CAD build for the part. Positions are in the model's coordinates, mm. Round coordinates to 2 decimals unless told otherwise and drop trailing zeros. Put each result on its own line as item: value. Start each with the question number.
Item 1: Mould opens along Z. For faces 1 (the flat face through (-6, 148, 10)), 2 (the cylindrical face through (0.54, 147.74, 2.44)), 3 (the flat face through (10, 148, 6)) say: released by +Z, released by -Z, zero draft, split by the parting line, or undercut.
Item 2: Drill centre lines: line 1 (Z direction, x = 0, y = 144); line 2 (X direction, y = 208, z = 7.5); line 3 (Z direction, x = 5.75, y = 162). Where is each one in solid material? Low to high. Write a range as from..to.
Item 3: Pin check, flat tips, straight feed: pin 1 Ø1.1 at (x, y) = (0.5, 116.5) entering from -Z; pin 2 Ø3 at (y, z) = (150, 0) entering from +X; pin 3 Ø4 at (x, y) = (0, 89) entering from +Z. Stop position of each tip, or through.
Autodesk Inventor part; units mm, degrees
ref_plane "Start Plane" through (0, 10, 0) normal (0, 1, 0) x (-1, 0, 0)
ref_plane "End Plane" through (0, 289.4, 0) normal (0, 1, 0) x (-1, 0, 0)
ref_plane "Work Plane5" through (9, 10, -660.4) normal (0, -1, 0) x (1, 0, 0)
ref_plane "Start Plane" through (0, 10, 0) normal (0, 1, 0) x (-1, 0, 0)
ref_plane "End Plane" through (0, 289.4, 0) normal (0, 1, 0) x (-1, 0, 0)
sketch "Sketch" plane through (0, 0, 0) normal (0, 1, 0) x (-1, 0, 0)
  line L0 (-1.7574, 4) -> (1.7574, 4)
  line L1 (4, 1.7574) -> (4, -1.7574)
  line L2 (1.7574, -4) -> (-1.7574, -4)
  line L3 (-4, -1.7574) -> (-4, 1.7574)
  line L4 (4.5858, -3.1716) -> (7.1464, -5.7322)
  line L5 (3.1716, -4.5858) -> (5.7322, -7.1464)
  line L6 (5.3787, -8) -> (3.5, -8)
  line L7 (3, -8.5) -> (3, -9.5)
  line L8 (3.5, -10) -> (9, -10)
  line L9 (10, -9) -> (10, -3.5)
  line L10 (9.5, -3) -> (8.5, -3)
  line L11 (8, -3.5) -> (8, -5.3787)
  line L12 (4, 0) -> (-4, 0) construction
  line L13 (0, -4) -> (0, 4) construction
  arc A0 (4, -1.7574) -> (4.5858, -3.1716) centre (6, -1.7574) ccw
  arc A1 (3.1716, -4.5858) -> (1.7574, -4) centre (1.7574, -6) ccw
  arc A2 (3.5, -8) -> (3, -8.5) centre (3.5, -8.5) ccw
  arc A3 (3, -9.5) -> (3.5, -10) centre (3.5, -9.5) ccw
  arc A4 (10, -3.5) -> (9.5, -3) centre (9.5, -3.5) ccw
  arc A5 (8.5, -3) -> (8, -3.5) centre (8.5, -3.5) ccw
  arc A6 (7.1464, -5.7322) -> (8, -5.3787) centre (7.5, -5.3787) ccw
  arc A7 (5.3787, -8) -> (5.7322, -7.1464) centre (5.3787, -7.5) ccw
  arc A8 (9, -10) -> (10, -9) centre (9, -9) ccw
  line L14 (-4.5858, -3.1716) -> (-7.1464, -5.7322)
  line L15 (-3.1716, -4.5858) -> (-5.7322, -7.1464)
  line L16 (-5.3787, -8) -> (-3.5, -8)
  line L17 (-3, -8.5) -> (-3, -9.5)
  line L18 (-3.5, -10) -> (-9, -10)
  line L19 (-10, -9) -> (-10, -3.5)
  line L20 (-9.5, -3) -> (-8.5, -3)
  line L21 (-8, -3.5) -> (-8, -5.3787)
  arc A9 (-4.5858, -3.1716) -> (-4, -1.7574) centre (-6, -1.7574) ccw
  arc A10 (-1.7574, -4) -> (-3.1716, -4.5858) centre (-1.7574, -6) ccw
  arc A11 (-3, -8.5) -> (-3.5, -8) centre (-3.5, -8.5) ccw
  arc A12 (-3.5, -10) -> (-3, -9.5) centre (-3.5, -9.5) ccw
  arc A13 (-9.5, -3) -> (-10, -3.5) centre (-9.5, -3.5) ccw
  arc A14 (-8, -3.5) -> (-8.5, -3) centre (-8.5, -3.5) ccw
  arc A15 (-8, -5.3787) -> (-7.1464, -5.7322) centre (-7.5, -5.3787) ccw
  arc A16 (-5.7322, -7.1464) -> (-5.3787, -8) centre (-5.3787, -7.5) ccw
  arc A17 (-10, -9) -> (-9, -10) centre (-9, -9) ccw
  line L22 (4.5858, 3.1716) -> (7.1464, 5.7322)
  line L23 (3.1716, 4.5858) -> (5.7322, 7.1464)
  line L24 (5.3787, 8) -> (3.5, 8)
  line L25 (3, 8.5) -> (3, 9.5)
  line L26 (3.5, 10) -> (9, 10)
  line L27 (10, 9) -> (10, 3.5)
  line L28 (9.5, 3) -> (8.5, 3)
  line L29 (8, 3.5) -> (8, 5.3787)
  arc A18 (4.5858, 3.1716) -> (4, 1.7574) centre (6, 1.7574) ccw
  arc A19 (1.7574, 4) -> (3.1716, 4.5858) centre (1.7574, 6) ccw
  arc A20 (3, 8.5) -> (3.5, 8) centre (3.5, 8.5) ccw
  arc A21 (3.5, 10) -> (3, 9.5) centre (3.5, 9.5) ccw
  arc A22 (9.5, 3) -> (10, 3.5) centre (9.5, 3.5) ccw
  arc A23 (8, 3.5) -> (8.5, 3) centre (8.5, 3.5) ccw
  arc A24 (8, 5.3787) -> (7.1464, 5.7322) centre (7.5, 5.3787) ccw
  arc A25 (5.7322, 7.1464) -> (5.3787, 8) centre (5.3787, 7.5) ccw
  arc A26 (10, 9) -> (9, 10) centre (9, 9) ccw
  line L30 (-10, 9) -> (-10, 3.5)
  arc A27 (-9, 10) -> (-10, 9) centre (-9, 9) ccw
  arc A28 (-10, 3.5) -> (-9.5, 3) centre (-9.5, 3.5) ccw
  line L31 (-9.5, 3) -> (-8.5, 3)
  arc A29 (-8.5, 3) -> (-8, 3.5) centre (-8.5, 3.5) ccw
  line L32 (-8, 3.5) -> (-8, 5.3787)
  arc A30 (-7.1464, 5.7322) -> (-8, 5.3787) centre (-7.5, 5.3787) ccw
  line L33 (-4.5858, 3.1716) -> (-7.1464, 5.7322)
  line L34 (-3.1716, 4.5858) -> (-5.7322, 7.1464)
  arc A31 (-3.1716, 4.5858) -> (-1.7574, 4) centre (-1.7574, 6) ccw
  arc A32 (-4, 1.7574) -> (-4.5858, 3.1716) centre (-6, 1.7574) ccw
  arc A33 (-5.3787, 8) -> (-5.7322, 7.1464) centre (-5.3787, 7.5) ccw
  line L35 (-5.3787, 8) -> (-3.5, 8)
  arc A34 (-3.5, 8) -> (-3, 8.5) centre (-3.5, 8.5) ccw
  line L36 (-3, 8.5) -> (-3, 9.5)
  arc A35 (-3, 9.5) -> (-3.5, 10) centre (-3.5, 9.5) ccw
  line L37 (-3.5, 10) -> (-9, 10)
  circle A36 centre (0, 0) radius 2.5
  point P0 (3, -8)
  point P1 (3, -10)
  point P2 (10, -10)
  dimension "d3" = 2
  dimension "d4" = 2
  dimension "d5" = 7
  dimension "d6" = 2
  dimension "d7" = 0.5
  dimension "d8" = 1
  dimension "d9" = 20
  dimension "d10" = 20
  dimension "d11" = 8
  dimension "d13" = 5
  dimension "d14" = 8
extrude "Body" add sketch "Sketch" along normal up to surface (279.4 mm away) from surface at 10
sketch "Sketch4" plane through (0, 0, 0) normal (0, 1, 0) x (-1, 0, 0)
  line L0 (0, 0) -> (10, 0)
ref_plane "Work Plane4" through (0, 0, 0) normal (0, 0, -1) x (-1, 0, 0)
sketch "Sketch5" plane through (0, 0, 0) normal (0, 0, -1) x (-1, 0, 0)
  line L0 (-2, 10) -> (12, 10)
  line L1 (-2, 289.4) -> (12, 289.4)
  dimension "d22" = 279.4
ref_plane "Work Plane5" through (9, 10, -660.4) normal (0, -1, 0) x (1, 0, 0)
split "Split1" plane through (9, 10, -660.4) removes the side toward (0, -1, 0)
ref_plane "Work Plane6" through (0, 289.4, 9) normal (0, 1, 0) x (1, 0, 0)
split "Split2" plane through (0, 289.4, 9) removes the side toward (0, 1, 0)
equation "\"d18\" = Length + G_OFFSET_END"
equation "\"G_L\" = d22"
properties part number "A3.3"
Output values:
1. face 1: released by +Z
1. face 2: undercut
1. face 3: zero draft
2. line 1: -4..-2.5, 2.5..4
2. line 2: -10..-5.88, 5.88..10
2. line 3: -10..-7.83, -7.17..-4.34, 4.34..7.17, 7.83..10
3. pin 1: z = -4
3. pin 2: x = 4
3. pin 3: z = 4.01
